Part model, mm, in its own coordinate system. A direction names the side the tool comes from. Round coordinates to 2 decimals unless told otherwise and drop trailing zeros. Loops run counter-clockwise (first coordinate to the right, second up) from the corner with the lowest first, then second, coordinate; pieces in that order, holes last. Notation, with made-up numbers: M 43,30 L 73,30 A30 cw 73,57 Z; hole C 50,65.25 d9. An arc over 180 degrees is marked long. Answer as CSV lines item,"result". Start each with the question number.
Item 1: Mould opens along Y. For faces 1 (the cylindrical face through (-0.59, 4.46, 6.72)), 2 (the cylindrical face through (-0.54, -2.44, 4.64)), 3 (the flat face through (2, -2, 0.4)), 4 (the flat face through (0, -5, 4.5)) say: pulls with the +Y half, pulls with the -Y half, needs draft (parallel to the pull), parting line crosses it, or undercut.
Item 2: Wall check: line 1 (Y direction, x = 0, z = 2.5); line 2 (Y direction, x = 0, z = 7); line 3 (Z direction, x = 5, y = 4.5). Give the ranges that are in metal, low to high.
Item 3: Drop flat-ended pins along their axis: pin 1 Ø1 at (x, z) = (3.5, 4) entering from -Y; pin 2 Ø3 at (y, z) = (4, 4) entering from -X; pin 3 Ø4 at (y, z) = (5.5, 7.5) entering from +X. Give the stop position or say it passes through.
Item 4: Band-saw the part on C-C (z = 3). Give the cut face in (x, y).
Item 5: Which spindle directions (+Z, -Z, +X, -X, +Y, -Y) get a long thin tool onto all of the face, cutting with end or side? Do faces 5 (the cylindrical face through (-0.59, 4.46, 0.2)), 6 (the flat face through (2, -2, 9)). Say none if no direction does.
Item 6: Band-saw the part on A-A (y = 0). Give the cut face in (x, z).
Item 7: Band-saw the part on D-D (y = 6). Give the cut face in (x, z), and give its area (3 significant figures).
```python
from build123d import *

# Parameters (mm, degrees)
F0_R     = 4.5
F0_R_2   = 2.5
F1_DEPTH = 9
F0_R_3   = 7.5
F2_DEPTH = 4.5
F3_DEPTH = 0.4


with BuildPart() as f1:
    # F0 (on Top) → F1 (new body)
    with BuildSketch(Plane.XY):
        Circle(F0_R)
        Circle(F0_R_2, mode=Mode.SUBTRACT)
    extrude(amount=F1_DEPTH)

    # F0 (on Top) → F2 (join)
    with BuildSketch(Plane.XY):
        Circle(F0_R_3)
        Circle(F0_R, mode=Mode.SUBTRACT)
    extrude(amount=F2_DEPTH)

    # F0 (on Top) → F3 (cut)
    with BuildSketch(Plane.XY):
        Circle(F0_R)
        Circle(F0_R_2, mode=Mode.SUBTRACT)
    extrude(amount=F3_DEPTH, mode=Mode.SUBTRACT)


solid = f1.part
```
Answer block:
1,face 1,"parting line crosses it"
1,face 2,"undercut"
1,face 3,"undercut"
1,face 4,"needs draft"
2,line 1,"y = -7.5 to -2.5, 2.5 to 7.5"
2,line 2,"y = -4.5 to -2.5, 2.5 to 4.5"
2,line 3,"z = 0 to 4.5"
3,pin 1,"stops at y = -6.87"
3,pin 2,"stops at x = -7.07"
3,pin 3,"stops at x = 2.83"
4,outline,"C 0,0 d15; hole C 0,0 d5"
5,face 5,"-Z"
5,face 6,"+Z, +X, -X, +Y, -Y"
6,outline,"M -7.5,0 L -4.5,0 L -4.5,0.4 L -2.5,0.4 L -2.5,9 L -4.5,9 L -4.5,4.5 L -7.5,4.5 Z; M 2.5,0.4 L 4.5,0.4 L 4.5,0 L 7.5,0 L 7.5,4.5 L 4.5,4.5 L 4.5,9 L 2.5,9 Z"
7,outline,"M -4.5,0 L 4.5,0 L 4.5,4.5 L -4.5,4.5 Z"
7,area,"40.5 mm^2"
